from build123d import *

# Parameters (mm, degrees)
SALIENTE_EXTRUIR1_DEPTH = 55
CROQUIS2_R              = 6.35
CORTAR_EXTRUIR1_DEPTH   = 55


with BuildPart() as part:
    # Croquis1 → Saliente-Extruir1 (new body)
    with BuildSketch(Plane.XY):
        with BuildLine():
            Line((0, 0), (0, -35))
            Line((0, -35), (20, -35))
            Line((20, -35), (20, 0))
            Line((20, 0), (20, 4.801960973))
            ThreePointArc((20, 4.801960973), (10, 25.930887204), (0, 4.801960973))
            Line((0, 4.801960973), (0, 0))
        make_face()
    extrude(amount=SALIENTE_EXTRUIR1_DEPTH)

    # Croquis2 → Cortar-Extruir1 (cut)
    with BuildSketch(Plane.XY.offset(55)):
        with Locations((10, 13)):
            Circle(CROQUIS2_R)
    extrude(amount=-CORTAR_EXTRUIR1_DEPTH, mode=Mode.SUBTRACT)


solid = part.part
Geometry check sheet. Reference: the model listing, model coordinates, mm. A direction names the side the tool comes from. Coordinates: 2 decimals unless noted, no trailing zeros. Order: outer loops, then holes, each group sorted by start corner. A loop starts at its lowest first (then second) coordinate and runs counter-clockwise, first axis right, second up. Notation, with made-up numbers: (89.25, -11.5) -> (101.25, -11.5) arc R10 cw to (101.25, -0.5) -> close; hole circle Ø3 at (39.5, -26.75). An arc over 180 degrees is marked (long way). Use a Markdown table: item, result. Add a question column.
1. Cross-section at C-C (z = 17). Enter the section's corners in (x, y), and give its area (3 significant figures).
2. Set-up check for faces 4 (the face through (10, -4, 55)), 5 (the face through (20, -15, 27)), 6 (the face through (0, -15, 27)): record each of +Z, -Z, +X, -X, +Y, -Y from which the full face is reachable in a straight line by a thin tool's end or side.
3. Mould release check, pull along Y, two halves, no side actions. Record for faces 1 (the face through (10, -35, 27)), 2 (the face through (5.32, 17.29, 27.88)), 3 (the face through (10.409, 25.924, 27.115)): pulls with the +Y half, pulls with the -Y half, needs draft (parallel to the pull), parting line crosses it, or undercut.
4. Cross-section at B-B (x = 10). Enter the section's corners in (y, z).
5. Go/stop test with flat-tipped pins: pin 1 Ø1.5 at (x, y) = (12, 3.5) entering from -Z; pin 2 Ø6 at (y, z) = (-21, 31) entering from +X; pin 3 Ø20 at (y, z) = (-11.5, 34) entering from -X; pin 4 Ø12 at (x, z) = (17.5, 30) entering from +Y. Record where each tip stops, or that it passes through.
6. Material ranges on L1, parallel to Y at x = 10.25, z = 3; L2, parallel to X at y = -29, z = 6; L3, parallel to X at y = 7.5, z = 29.5, recorded low to high.
7. Cross-section at A-A (y = 13). Enter the section's corners in (x, z), and give its area (3 significant figures).
8. Cross-section at D-D (y = -7). Enter the section's corners in (x, z).
Filled sheet:
| question | item | result |
|---|---|---|
| 1 | outline | (0, -35) -> (20, -35) -> (20, 4.8) arc R12.93 ccw (long way) to (0, 4.8) -> close; hole circle Ø12.7 at (10, 13) |
| 1 | area | 1,130 mm2 |
| 2 | face 4 | +Z, +X, -X, +Y, -Y |
| 2 | face 5 | +Z, -Z, +X, -Y |
| 2 | face 6 | +Z, -Z, -X, -Y |
| 3 | face 1 | pulls with the -Y half |
| 3 | face 2 | undercut |
| 3 | face 3 | parting line crosses it |
| 4 | outline | (-35, 0) -> (6.65, 0) -> (6.65, 55) -> (-35, 55) -> close; (19.35, 0) -> (25.93, 0) -> (25.93, 55) -> (19.35, 55) -> close |
| 5 | pin 1 | z = 0 |
| 5 | pin 2 | x = 20 |
| 5 | pin 3 | x = 0 |
| 5 | pin 4 | y = 25.84 |
| 6 | L1 | -35 to 6.65, 19.35 to 25.93 |
| 6 | L2 | 0 to 20 |
| 6 | L3 | -1.7 to 6.83, 13.17 to 21.7 |
| 7 | outline | (-2.93, 0) -> (3.65, 0) -> (3.65, 55) -> (-2.93, 55) -> close; (16.35, 0) -> (22.93, 0) -> (22.93, 55) -> (16.35, 55) -> close |
| 7 | area | 724 mm2 |
| 8 | outline | (0, 0) -> (20, 0) -> (20, 55) -> (0, 55) -> close |
